Geometry: final body of the model. Coordinates: model frame, mm. A direction names the side the tool comes from. Round coordinates to 2 decimals unless told otherwise and drop trailing zeros. Loops run counter-clockwise (first coordinate to the right, second up) from the corner with the lowest first, then second, coordinate; pieces in that order, holes last. Notation, with made-up numbers: (51, -4.5) - (60, -4.5) arc R25 ccw to (60, 34.5) - close; hole circle Ø6 at (68, 69). An arc over 180 degrees is marked (long way). Write item = value, one per line. Start each with the question number.
Item 1: Access query for faces 3 (the flat face through (955, 1027.342, 1049)), 4 (the flat face through (984.363, 1020, 1051)), 5 (the flat face through (929.263, 1001, 1053)), 6 (the flat face through (885, 1011.157, 1048)). Directions: +Z, -Z, +X, -X, +Y, -Y. A direction counts if a zero-diameter tool reaches every point of the face in a straight line with its end or side. Return the directions, or none.
Item 2: First-contact query: pin 1 (12 mm diameter, centred on x = 938, y = 1005.5, fed in from -Z); pin 2 (1 mm diameter, centred on x = 926, z = 1049.5, fed in from -Y); pin 3 (1.5 mm diameter, centred on x = 917, y = 1038, fed in from -Z). Flat tips, straight axial feed; report the tip coordinate or a pass-through.
Item 3: Draft query along Y for faces 1 (the flat face through (944.475, 1019, 1050)), 2 (the flat face through (885, 1013, 1046.483)). Return one class per face: pulls with the +Y half, pulls with the -Y half, needs draft (parallel to the pull), parting line crosses it, or undercut.
Item 4: Section B-B (x = 899). Return loops of the section in (y, z), plus the area to 3 significant figures.
Item 5: Line query: line 1 (Y direction, x = 960, z = 1051.75); line 2 (X direction, y = 999.5, z = 1052.5); line 3 (Y direction, x = 916, z = 1051.5). Output: solid intervals per line, ascending. Write a range as from..to.
Item 6: Section A-A (y = 1002.5). Return loops of the section in (x, z), plus the area to 3 significant figures.
from build123d import *

# Parameters (mm, degrees)
SKETCH_1_W           = 99.974800609
SKETCH_1_H           = 51.97470409
EXTRUDE_1_DEPTH      = 8.6
SKETCH_2_W           = 95.974800609
SKETCH_2_H           = 47.97470409
CUT_EXTRUDE_1_DEPTH  = 4
SKETCH_3_W           = 2
SKETCH_3_H           = 10
SKETCH_3_H_2         = 9.97470409
CUT_EXTRUDE_2_DEPTH  = 3.35
SKETCH_4_R           = 1.1
SKETCH_4_W           = 38.392586289
SKETCH_4_H           = 7.4
SKETCH_4_W_2         = 5.95
SKETCH_4_H_2         = 5.95
CUT_EXTRUDE_3_DEPTH  = 1437.448457956
SKETCH_6_W           = 6.76
SKETCH_6_H           = 6.795709929
CUT_EXTRUDE_4_DEPTH  = 4.5
FILLET_1_R           = 3
FILLET_3_R           = 2
SKETCH_12_W          = 9.000025401
SKETCH_12_H          = 9.0000508
EXTRUDE_3_DEPTH      = 2.7
SKETCH_13_W          = 16.992125984
SKETCH_13_H          = 17.047314393
EXTRUDE_4_DEPTH      = 1.9
SKETCH_7_W           = 53.6
SKETCH_7_H           = 10.97470409
CUT_EXTRUDE_14_DEPTH = 4
FILLET_7_R           = 2
FILLET_8_R           = 1
SKETCH_14_W          = 2.323736835
SKETCH_14_H          = 6.8
CUT_EXTRUDE_15_DEPTH = 2


with BuildPart() as part:
    # 草图1 → 凸台-拉伸1 (new body)
    with BuildSketch(Plane.XY.offset(1046.483288979)):
        with Locations((934.375963031, 1020.144466268)):
            Rectangle(SKETCH_1_W, SKETCH_1_H)
    extrude(amount=EXTRUDE_1_DEPTH)

    # 草图2 → 切除-拉伸1 (cut)
    with BuildSketch(Plane(origin=(0, 0, 1046.483288979), x_dir=(-1, 0, 0), z_dir=(0, 0, -1))):
        with Locations((-934.375963031, 1020.144466268)):
            Rectangle(SKETCH_2_W, SKETCH_2_H)
    extrude(amount=-CUT_EXTRUDE_1_DEPTH, mode=Mode.SUBTRACT)

    # 草图3 → 切除-拉伸2 (cut)
    with BuildSketch(Plane(origin=(0, 0, 1046.483288979), x_dir=(-1, 0, 0), z_dir=(0, 0, -1))):
        with Locations((-885.388562726, 1034.131818313)):
            Rectangle(SKETCH_3_W, SKETCH_3_H)
        with Locations((-885.388562726, 1020.144466268)):
            Rectangle(SKETCH_3_W, SKETCH_3_H_2)
        with Locations((-885.388562726, 1006.157114223)):
            Rectangle(SKETCH_3_W, SKETCH_3_H)
    extrude(amount=-CUT_EXTRUDE_2_DEPTH, mode=Mode.SUBTRACT)

    # 草图4 → 切除-拉伸3 (cut, through all)
    with BuildSketch(Plane(origin=(0, 0, 1050.483288979), x_dir=(-1, 0, 0), z_dir=(0, 0, -1))):
        with Locations((-920.388562726, 1041.631818313)):
            Circle(SKETCH_4_R)
        with Locations((-920.388562726, 998.657114223)):
            Circle(SKETCH_4_R)
        with Locations((-972.363363335, 998.657114223)):
            Circle(SKETCH_4_R)
        with Locations((-972.363363335, 1041.631818313)):
            Circle(SKETCH_4_R)
        with Locations((-949.933821712, 1001.144429438)):
            Rectangle(SKETCH_4_W, SKETCH_4_H)
        with Locations((-977.376048121, 1035.144495478)):
            Rectangle(SKETCH_4_W_2, SKETCH_4_H_2)
    extrude(amount=-CUT_EXTRUDE_3_DEPTH, mode=Mode.SUBTRACT)

    # 草图6 → 切除-拉伸4 (cut)
    with BuildSketch(Plane(origin=(0, 0, 1046.483288979), x_dir=(-1, 0, 0), z_dir=(0, 0, -1))):
        with Locations((-926.946347841, 997.554969188)):
            Rectangle(SKETCH_6_W, SKETCH_6_H)
    extrude(amount=-CUT_EXTRUDE_4_DEPTH, mode=Mode.SUBTRACT)

    # 圆角1
    fillet_1_edges = [part.edges().sort_by_distance(p)[0] for p in [
        (884.388562726, 1046.131818313, 1050.783288979),
        (984.363363335, 1046.131818313, 1050.783288979),
        (984.363363335, 994.157114223, 1050.783288979),
        (884.388562726, 994.157114223, 1050.783288979),
    ]]
    fillet(fillet_1_edges, radius=FILLET_1_R)

    # 圆角3
    fillet_3_edges = [part.edges().sort_by_distance(p)[0] for p in [
        (980.351048121, 1032.169495478, 1052.783288979),
        (980.351048121, 1038.119495478, 1052.783288979),
        (974.401048121, 1038.119495478, 1052.783288979),
        (974.401048121, 1032.169495478, 1052.783288979),
    ]]
    fillet(fillet_3_edges, radius=FILLET_3_R)

    # 草图12 → 凸台-拉伸3 (add)
    with BuildSketch(Plane(origin=(0, 0, 1050.483288979), x_dir=(-1, 0, 0), z_dir=(0, 0, -1))):
        with Locations((-955.369926709, 1022.842410134)):
            Rectangle(SKETCH_12_W, SKETCH_12_H)
    extrude(amount=EXTRUDE_3_DEPTH)

    # 草图13 → 凸台-拉伸4 (add)
    with BuildSketch(Plane(origin=(0, 0, 1050.483288979), x_dir=(-1, 0, 0), z_dir=(0, 0, -1))):
        with Locations((-935.979052947, 1018.778239857)):
            Rectangle(SKETCH_13_W, SKETCH_13_H)
    extrude(amount=EXTRUDE_4_DEPTH)

    # 草图7 → 切除-拉伸14 (cut)
    with BuildSketch(Plane.XY.offset(1055.083288979)):
        Polygon((885.888562726, 1019.831818313), (982.863363335, 1019.831818313), (982.863363335, 1008.131818313), (927.763363335, 1008.131818313), (927.763363335, 1006.631818313), (927.763363335, 995.657114223), (885.888562726, 995.657114223), align=None)
        Polygon((934.163363335, 1044.631818313), (934.163363335, 1033.131818313), (935.663363335, 1033.131818313), (935.663363335, 1044.631818313), (982.863363335, 1044.631818313), (982.863363335, 1021.331818313), (963.463363335, 1021.331818313), (963.463363335, 1032.731818313), (943.963363335, 1032.731818313), (943.963363335, 1031.231818313), (961.963363335, 1031.231818313), (961.963363335, 1021.331818313), (927.563363335, 1021.331818313), (927.563363335, 1032.811818313), (904.363363335, 1032.811818313), (904.363363335, 1044.631818313), align=None)
        with Locations((956.063363335, 1001.144466268)):
            Rectangle(SKETCH_7_W, SKETCH_7_H)
        Polygon((926.063363335, 1021.331818313), (926.063363335, 1031.311818313), (902.863363335, 1031.311818313), (902.863363335, 1044.631818313), (885.888562726, 1044.631818313), (885.888562726, 1021.331818313), align=None)
    extrude(amount=-CUT_EXTRUDE_14_DEPTH, mode=Mode.SUBTRACT)

    # 圆角7
    fillet_7_edges = [part.edges().sort_by_distance(p)[0] for p in [
        (923.566347841, 1000.952824152, 1050.733288979),
        (930.326347841, 1000.952824152, 1050.733288979),
        (982.363363335, 996.157114223, 1048.483288979),
        (982.363363335, 1044.131818313, 1048.483288979),
        (886.388562726, 1044.131818313, 1048.483288979),
        (886.388562726, 996.157114223, 1048.483288979),
        (982.863363335, 995.657114223, 1053.083288979),
        (929.263363335, 995.657114223, 1053.083288979),
        (929.263363335, 1006.631818313, 1053.083288979),
        (982.863363335, 1006.631818313, 1053.083288979),
        (961.963363335, 1021.331818313, 1053.083288979),
        (927.563363335, 1021.331818313, 1053.083288979),
        (927.563363335, 1032.811818313, 1053.083288979),
        (904.363363335, 1032.811818313, 1053.083288979),
        (904.363363335, 1044.631818313, 1053.083288979),
        (934.163363335, 1044.631818313, 1053.083288979),
        (935.663363335, 1044.631818313, 1053.083288979),
        (982.863363335, 1044.631818313, 1053.083288979),
        (982.863363335, 1021.331818313, 1053.083288979),
        (963.463363335, 1021.331818313, 1053.083288979),
        (963.463363335, 1032.731818313, 1053.083288979),
        (961.963363335, 1031.231818313, 1053.083288979),
        (885.888562726, 1021.331818313, 1053.083288979),
        (885.888562726, 1044.631818313, 1053.083288979),
        (902.863363335, 1044.631818313, 1053.083288979),
        (902.863363335, 1031.311818313, 1053.083288979),
        (926.063363335, 1031.311818313, 1053.083288979),
        (926.063363335, 1021.331818313, 1053.083288979),
        (927.763363335, 995.657114223, 1053.083288979),
        (885.888562726, 995.657114223, 1053.083288979),
        (885.888562726, 1019.831818313, 1053.083288979),
        (982.863363335, 1019.831818313, 1053.083288979),
        (982.863363335, 1008.131818313, 1053.083288979),
        (927.763363335, 1008.131818313, 1053.083288979),
    ]]
    fillet(fillet_7_edges, radius=FILLET_7_R)

    # 圆角8
    fillet_8_edges = [part.edges().sort_by_distance(p)[0] for p in [
        (930.737528567, 997.444429438, 1050.783288979),
        (969.130114856, 997.444429438, 1050.783288979),
        (930.737528567, 1004.844429438, 1050.783288979),
        (969.130114856, 1004.844429438, 1050.783288979),
    ]]
    fillet(fillet_8_edges, radius=FILLET_8_R)

    # 草图14 → 切除-拉伸15 (cut)
    with BuildSketch(Plane.XY.offset(1055.083288979)):
        with Locations((983.201494917, 1013.231818313)):
            Rectangle(SKETCH_14_W, SKETCH_14_H)
    extrude(amount=-CUT_EXTRUDE_15_DEPTH, mode=Mode.SUBTRACT)


solid = part.part
Taken from the geometry:
q1.face_3 = -Z
q1.face_4 = +Z, -Z, +X, +Y, -Y
q1.face_5 = +Z
q1.face_6 = -Z, -X
q2.pin_1 = 1048.58
q2.pin_2 = 1044.13
q2.pin_3 = 1050.48
q3.face_1 = undercut
q3.face_2 = needs draft
q4.outline = (994.16, 1046.48) - (996.16, 1046.48) - (996.16, 1050.48) - (1044.13, 1050.48) - (1044.13, 1046.48) - (1046.13, 1046.48) - (1046.13, 1055.08) - (1044.63, 1055.08) - (1044.63, 1051.08) - (1021.33, 1051.08) - (1021.33, 1055.08) - (1019.83, 1055.08) - (1019.83, 1051.08) - (995.66, 1051.08) - (995.66, 1055.08) - (994.16, 1055.08) - close
q4.area = 65.2 mm^2
q5.line_1 = 994.16..995.66, 1006.63..1008.13, 1019.83..1021.33, 1031.23..1032.73, 1044.63..1046.13
q5.line_2 = 884.39..885.89, 927.76..929.26, 982.86..984.36
q5.line_3 = 994.16..995.66, 1019.83..1021.33, 1031.31..1032.81, 1044.63..1046.13
q6.outline = (884.39, 1049.83) - (886.39, 1049.83) - (886.39, 1050.48) - (930.74, 1050.48) - (930.74, 1051.08) - (929.26, 1051.08) - (929.26, 1055.08) - (927.76, 1055.08) - (927.76, 1051.08) - (885.89, 1051.08) - (885.89, 1055.08) - (884.39, 1055.08) - close; (969.13, 1050.48) - (982.36, 1050.48) - (982.36, 1046.48) - (984.36, 1046.48) - (984.36, 1055.08) - (982.86, 1055.08) - (982.86, 1051.08) - (969.13, 1051.08) - close
q6.area = 64.2 mm^2
